Build history of the part. All positions in model axes, mm. Give positions to 0.01 mm unless a question says otherwise; leave off trailing zeros. Order: outer loops, then holes, each group sorted by start corner. A loop starts at its lowest first (then second) coordinate and runs counter-clockwise, first axis right, second up. Notation, with made-up numbers: (-15.5, 5.25) - (7.5, 5.25) arc R26 ccw to (7.5, 34.25) - close; hole circle Ø11 at (-27.75, 79.5). An arc over 180 degrees is marked (long way). One line per item, written item: value.
```python
from build123d import *

# Parameters (mm, degrees)
SKETCH1_W           = 93
SKETCH1_H           = 25
BOSS_EXTRUDE1_DEPTH = 18.5
FILLET1_R           = 2
FILLET2_R           = 2
BOSS_EXTRUDE2_DEPTH = 0.01
SKETCH4_RX          = 13.895867653
SKETCH4_RY          = 6.24610939
CUT_EXTRUDE1_DEPTH  = 0.1
SKETCH5_RX          = 21.704276093
SKETCH5_RY          = 7.058205551
CUT_EXTRUDE2_DEPTH  = 0.1


with BuildPart() as part:
    # Sketch1 → Boss-Extrude1 (new body)
    with BuildSketch(Plane(origin=(0, 0, 0), x_dir=(1, 0, 0), z_dir=(0, 1, 0))):
        Rectangle(SKETCH1_W, SKETCH1_H)
    extrude(amount=BOSS_EXTRUDE1_DEPTH)

    # Fillet1
    fillet1_edges = [part.edges().sort_by_distance(p)[0] for p in [
        (-46.5, 18.5, 0),
        (46.5, 18.5, 0),
        (-46.5, 0, 0),
        (46.5, 0, 0),
    ]]
    fillet(fillet1_edges, radius=FILLET1_R)

    # Fillet2
    # the kernel refuses this fillet: 2 mm, written as the material it takes off along each edge
    with BuildSketch(Plane(origin=(-49.5, 18.5, -12.5), x_dir=(0, -1, 0), z_dir=(1, 0, 0))) as fillet2_piece_1:
        with BuildLine():
            CenterArc((FILLET2_R, -FILLET2_R), FILLET2_R, 90, 90)
            Line((0, -FILLET2_R), (0, 0))
            Line((0, 0), (FILLET2_R, 0))
        make_face()
    extrude(amount=94, mode=Mode.SUBTRACT)
    with BuildSketch(Plane(origin=(44.5, 18.5, 12.5), x_dir=(0, 0, -1), z_dir=(-1, 0, 0))) as fillet2_piece_2:
        with BuildLine():
            CenterArc((FILLET2_R, FILLET2_R), FILLET2_R, 180, 90)
            Line((0, FILLET2_R), (0, 0))
            Line((0, 0), (FILLET2_R, 0))
        make_face()
    extrude(amount=89, mode=Mode.SUBTRACT)
    with BuildSketch(Plane(origin=(44.5, 0, 12.5), x_dir=(0, 0, -1), z_dir=(-1, 0, 0))) as fillet2_piece_3:
        with BuildLine():
            CenterArc((FILLET2_R, -FILLET2_R), FILLET2_R, 90, 90)
            Line((0, -FILLET2_R), (0, 0))
            Line((0, 0), (FILLET2_R, 0))
        make_face()
    extrude(amount=89, mode=Mode.SUBTRACT)
    with BuildSketch(Plane(origin=(46.5, 2, 12.5), x_dir=(0, 0, -1), z_dir=(0, 1, 0)), Plane(origin=(46.5, 2, -12.5), x_dir=(-1, 0, 0), z_dir=(0, 1, 0))) as fillet2_piece_4:
        with BuildLine():
            CenterArc((FILLET2_R, FILLET2_R), FILLET2_R, 180, 90)
            Line((0, FILLET2_R), (0, 0))
            Line((0, 0), (FILLET2_R, 0))
        make_face()
    extrude(amount=14.5, mode=Mode.SUBTRACT)
    with BuildSketch(Plane(origin=(-46.5, 2, 12.5), x_dir=(0, 0, -1), z_dir=(0, 1, 0))) as fillet2_piece_5:
        with BuildLine():
            CenterArc((FILLET2_R, -FILLET2_R), FILLET2_R, 90, 90)
            Line((0, -FILLET2_R), (0, 0))
            Line((0, 0), (FILLET2_R, 0))
        make_face()
    extrude(amount=14.5, mode=Mode.SUBTRACT)
    with BuildSketch(Plane(origin=(44.5, 16.5, 12.5), x_dir=(1, 0, 0), z_dir=(0, -1, 0))) as fillet2_piece_6:
        with BuildLine():
            CenterArc((2 - FILLET2_R, -FILLET2_R), FILLET2_R, 0, 90)
            Line((2 - FILLET2_R, 0), (2, 0))
            Line((2, 0), (2, -FILLET2_R))
        make_face()
    revolve(axis=Axis((44.5, 16.5, 12.5), (0, 0, 1)), revolution_arc=90, mode=Mode.SUBTRACT)
    with BuildSketch(Plane(origin=(44.5, 2, 12.5), x_dir=(1, 0, 0), z_dir=(0, 1, 0))) as fillet2_piece_7:
        with BuildLine():
            CenterArc((2 - FILLET2_R, FILLET2_R), FILLET2_R, 270, 90)
            Line((2 - FILLET2_R, 0), (2, 0))
            Line((2, 0), (2, FILLET2_R))
        make_face()
    revolve(axis=Axis((44.5, 2, 12.5), (0, 0, -1)), revolution_arc=90, mode=Mode.SUBTRACT)
    with BuildSketch(Plane(origin=(-44.5, 2, 12.5), x_dir=(-1, 0, 0), z_dir=(0, 1, 0))) as fillet2_piece_8:
        with BuildLine():
            CenterArc((2 - FILLET2_R, -FILLET2_R), FILLET2_R, 0, 90)
            Line((2 - FILLET2_R, 0), (2, 0))
            Line((2, 0), (2, -FILLET2_R))
        make_face()
    revolve(axis=Axis((-44.5, 2, 12.5), (0, 0, 1)), revolution_arc=90, mode=Mode.SUBTRACT)
    with BuildSketch(Plane(origin=(-44.5, 16.5, 12.5), x_dir=(-1, 0, 0), z_dir=(0, -1, 0))) as fillet2_piece_9:
        with BuildLine():
            CenterArc((2 - FILLET2_R, FILLET2_R), FILLET2_R, 270, 90)
            Line((2 - FILLET2_R, 0), (2, 0))
            Line((2, 0), (2, FILLET2_R))
        make_face()
    revolve(axis=Axis((-44.5, 16.5, 12.5), (0, 0, -1)), revolution_arc=90, mode=Mode.SUBTRACT)
    with BuildSketch(Plane(origin=(-49.5, 0, -12.5), x_dir=(0, 1, 0), z_dir=(1, 0, 0))) as fillet2_piece_10:
        with BuildLine():
            CenterArc((FILLET2_R, FILLET2_R), FILLET2_R, 180, 90)
            Line((0, FILLET2_R), (0, 0))
            Line((0, 0), (FILLET2_R, 0))
        make_face()
    extrude(amount=94, mode=Mode.SUBTRACT)
    with BuildSketch(Plane(origin=(44.5, 16.5, -12.5), x_dir=(1, 0, 0), z_dir=(0, -1, 0))) as fillet2_piece_11:
        with BuildLine():
            CenterArc((2 - FILLET2_R, FILLET2_R), FILLET2_R, 270, 90)
            Line((2, FILLET2_R), (2, 0))
            Line((2, 0), (2 - FILLET2_R, 0))
        make_face()
    revolve(axis=Axis((44.5, 16.5, -12.5), (0, 0, 1)), revolution_arc=90, mode=Mode.SUBTRACT)
    with BuildSketch(Plane(origin=(44.5, 2, -12.5), x_dir=(1, 0, 0), z_dir=(0, 1, 0))) as fillet2_piece_12:
        with BuildLine():
            CenterArc((2 - FILLET2_R, -FILLET2_R), FILLET2_R, 0, 90)
            Line((2, -FILLET2_R), (2, 0))
            Line((2, 0), (2 - FILLET2_R, 0))
        make_face()
    revolve(axis=Axis((44.5, 2, -12.5), (0, 0, -1)), revolution_arc=90, mode=Mode.SUBTRACT)

    # Sketch3 → Boss-Extrude2 (add)
    with BuildSketch(Plane(origin=(0, 18.5, 0), x_dir=(-1, 0, 0), z_dir=(0, 1, 0))):
        with BuildLine():
            Line((-32.5, 11), (32.5, 11))
            ThreePointArc((32.5, 11), (33.560660172, 10.560660172), (34, 9.5))
            Line((34, 9.5), (34, -9.5))
            ThreePointArc((34, -9.5), (33.560660172, -10.560660172), (32.5, -11))
            Line((32.5, -11), (-32.5, -11))
            ThreePointArc((-32.5, -11), (-33.560660172, -10.560660172), (-34, -9.5))
            Line((-34, -9.5), (-34, 9.5))
            ThreePointArc((-34, 9.5), (-33.560660172, 10.560660172), (-32.5, 11))
        make_face()
    extrude(amount=BOSS_EXTRUDE2_DEPTH)

    # Sketch4 → Cut-Extrude1 (cut)
    with BuildSketch(Plane(origin=(46.5, 0, 0), x_dir=(0, 0, -1), z_dir=(1, 0, 0))):
        with Locations(Location((0, 9.25), (0, 0, 180))):
            Ellipse(SKETCH4_RX, SKETCH4_RY)
    extrude(amount=-CUT_EXTRUDE1_DEPTH, mode=Mode.SUBTRACT)

    # Sketch5 → Cut-Extrude2 (cut)
    with BuildSketch(Plane.ZY.offset(46.5)):
        with Locations(Location((-7.207732319, 9.25), (0, 0, 180))):
            Ellipse(SKETCH5_RX, SKETCH5_RY)
    extrude(amount=-CUT_EXTRUDE2_DEPTH, mode=Mode.SUBTRACT)


solid = part.part
```
(1) Slice it at A-A, the plane y = 17.5. Give the cut face in (x, z), and give its area (3 significant figures).
Completed:
outline: (-46.23, -12.23) - (44.5, -12.23) arc R1.73 ccw to (46.23, -10.5) - (46.23, 10.5) arc R1.73 ccw to (44.5, 12.23) - (-44.5, 12.23) arc R1.73 ccw to (-46.23, 10.5) - close
area: 2,260 mm²
(2) Pull direction Y, two halves, no side cores. Call faces 1 (the face through (45.7, 9.1, -12.1)), 2 (the face through (-39, 18.5, 0)), 3 (the face through (-46.4, 9, -1)): +Y half, -Y half, draft (parallel to the pull), parting line (faces both ways), or undercut.
Completed:
face 1: draft
face 2: +Y half
face 3: undercut
(3) Pin check, flat tips, straight feed: P1, Ø6, axis at y = 10, z = 5, coming from the +X side; P2, Ø5.5, axis at x = 40.5, z = 4, coming from the +Y side; P3, Ø1.5, axis at y = 4.5, z = 5, coming from the -X side. Stop position of each tip, or through.
Completed:
P1: x = 46.4
P2: y = 18.5
P3: x = -46.4
(4) Drill centre lines: line 1 (X direction, y = 4.25, z = 7.25); line 2 (Y direction, x = -41, z = -1); line 3 (Z direction, x = 1, y = 16.75). Where is each one in solid material? Low to high.
Completed:
line 1: -46.4 to 46.4
line 2: 0 to 18.5
line 3: -12.48 to 12.48
